Build history of the part. All positions in model axes, mm. Round coordinates to 2 decimals unless told otherwise and drop trailing zeros. Order: outer loops, then holes, each group sorted by start corner. A loop starts at its lowest first (then second) coordinate and runs counter-clockwise, first axis right, second up. Notation, with made-up numbers: (26, 11) - (83, 11) arc R19 ccw to (83, 31) - close; hole circle Ø7 at (-8, 4). An arc over 180 degrees is marked (long way). One line per question, with ' | ' between items. Start each with the question number.
from build123d import *

# Parameters (mm, degrees)
SKETCH1_R           = 7.5
BOSS_EXTRUDE1_DEPTH = 15


with BuildPart() as part:
    # Sketch1 → Boss-Extrude1 (new body)
    with BuildSketch(Plane.XZ):
        with BuildLine():
            Line((-70, 13), (70, 13))
            ThreePointArc((70, 13), (83, 0), (70, -13))
            Line((70, -13), (-70, -13))
            ThreePointArc((-70, -13), (-83, 0), (-70, 13))
        make_face()
        with Locations(Location((-70, 0, 0), (0, 0, 90))):
            Circle(SKETCH1_R, mode=Mode.SUBTRACT)
        with Locations(Location((70, 0, 0), (0, 0, 90))):
            Circle(SKETCH1_R, mode=Mode.SUBTRACT)
    extrude(amount=-BOSS_EXTRUDE1_DEPTH)


solid = part.part
Item 1: Slice it at B-B (y = 5). Write the cut outline in (x, z).
Item 2: Slice it at A-A (z = 0). Write the cut outline in (x, y), plus the area to 3 significant figures.
Item 3: Pull direction X, two halves, no side cores. Call faces 1 (the face through (83, 7, 0)), 2 (the face through (1, 0, 0)), 3 (the face through (-62.68, 7.4, -1.63)): released by +X, released by -X, zero draft, split by the parting line, or undercut.
Item 4: Slice it at D-D (z = -11). Write the cut outline in (x, y).
Item 5: Wall check: line 1 along X through (y, z) = (9.5, 0); line 2 along Z through (x, y) = (-70, 7.5); line 3 along X through (y, z) = (5.75, -5). Give the ranges that are in metal, low to high. Write a range as [from, to].
Item 6: Pin check, flat tips, straight feed: pin 1 (8 mm diameter, centred on y = 10.5, z = 8, fed in from +X); pin 2 (4 mm diameter, centred on y = 10.5, z = -6.5, fed in from -X); pin 3 (1.5 mm diameter, centred on y = 7.5, z = 9.5, fed in from +X). Stop position of each tip, or through.
Item 7: Slice it at C-C (z = 9). Write the cut outline in (x, y).
A:
1) outline: (-70, -13) - (70, -13) arc R13 ccw to (70, 13) - (-70, 13) arc R13 ccw to start; hole circle Ø15 at (-70, 0); hole circle Ø15 at (70, 0)
2) outline: (-83, 0) - (-77.5, 0) - (-77.5, 15) - (-83, 15) - close; (-62.5, 0) - (62.5, 0) - (62.5, 15) - (-62.5, 15) - close; (77.5, 0) - (83, 0) - (83, 15) - (77.5, 15) - close | area: 2,040 mm^2
3) face 1: released by +X | face 2: zero draft | face 3: undercut
4) outline: (-76.93, 0) - (76.93, 0) - (76.93, 15) - (-76.93, 15) - close
5) line 1: [-83, -77.5], [-62.5, 62.5], [77.5, 83] | line 2: [-13, -7.5], [7.5, 13] | line 3: [-82, -75.59], [-64.41, 64.41], [75.59, 82]
6) pin 1: x = 82.37 | pin 2: x = -82.2 | pin 3: x = 79.61
7) outline: (-79.38, 0) - (79.38, 0) - (79.38, 15) - (-79.38, 15) - close
